from build123d import *

# Parameters (mm, degrees)
F0_W      = 19.05
F0_H      = 19.05
F1_DEPTH  = 19.05
F2_R      = 7.62
F3_DEPTH  = 0.889
F4_R      = 0.999998
F5_DEPTH  = 4.7752
F6_R      = 7.62
F7_DEPTH  = 15.5702
F9_DEPTH  = 6.8573073039
F10_R     = 1.5875
F10_R_2   = 1.9939
F11_DEPTH = 3.4808
F12_R     = 0.999998
F13_DEPTH = 4.7752


with BuildPart() as f1:
    # F0 (on Top) → F1 (new body)
    with BuildSketch(Plane.XY):
        Rectangle(F0_W, F0_H)
    extrude(amount=F1_DEPTH)

    # F2 (on face) → F3 (cut)
    with BuildSketch(Plane.XY.offset(19.05)):
        Circle(F2_R)
        with BuildLine():
            ThreePointArc((4.9464736177, -2.544585921), (-5.5626, 0), (4.9464736177, 2.544585921))
            ThreePointArc((4.9464736177, 2.544585921), (6.5611449159, 1.7206267132), (7.1316849154, 0))
            ThreePointArc((7.1316849154, 0), (6.5611449159, -1.7206267132), (4.9464736177, -2.544585921))
        make_face(mode=Mode.SUBTRACT)
    extrude(amount=-F3_DEPTH, mode=Mode.SUBTRACT)

    # F4 (on face) → F5 (cut)
    with BuildSketch(Plane.XY.offset(19.05)):
        with Locations((-5.7912, -7.874)):
            Circle(F4_R)
        with Locations((5.7912, -7.874)):
            Circle(F4_R)
        with Locations((6.985, 7.747)):
            Circle(F4_R)
        with Locations((-6.985, 7.747)):
            Circle(F4_R)
    extrude(amount=-F5_DEPTH, mode=Mode.SUBTRACT)

    # F6 (on face) → F7 (cut)
    with BuildSketch(Plane.XZ.offset(9.525)):
        with Locations((0, 9.525)):
            Circle(F6_R)
    extrude(amount=-F7_DEPTH, mode=Mode.SUBTRACT)

    # F8 (on face) → F9 (cut, through all)
    with BuildSketch(Plane.XY.offset(19.05)):
        with BuildLine():
            ThreePointArc((4.9464736177, 2.544585921), (-5.5626, 0), (4.9464736177, -2.544585921))
            ThreePointArc((4.9464736177, -2.544585921), (6.5611449159, -1.7206267132), (7.1316849154, 0))
            ThreePointArc((7.1316849154, 0), (6.5611449159, 1.7206267132), (4.9464736177, 2.544585921))
        make_face()
    extrude(amount=-F9_DEPTH, mode=Mode.SUBTRACT)

    # F10 (on face) → F11 (cut, through all)
    with BuildSketch(Plane.XZ.offset(-6.0452)):
        with Locations((0, 9.525)):
            Circle(F10_R)
        with Locations((-4.7752, 9.525)):
            Circle(F10_R_2)
    extrude(amount=-F11_DEPTH, mode=Mode.SUBTRACT)

    # F12 (on face) → F13 (cut)
    with BuildSketch(Plane.XZ.offset(9.525)):
        with Locations((-8.001, 16.51)):
            Circle(F12_R)
        with Locations((8.001, 16.51)):
            Circle(F12_R)
        with Locations((-6.985, 2.54)):
            Circle(F12_R)
        with Locations((6.985, 2.54)):
            Circle(F12_R)
    extrude(amount=-F13_DEPTH, mode=Mode.SUBTRACT)


solid = f1.part
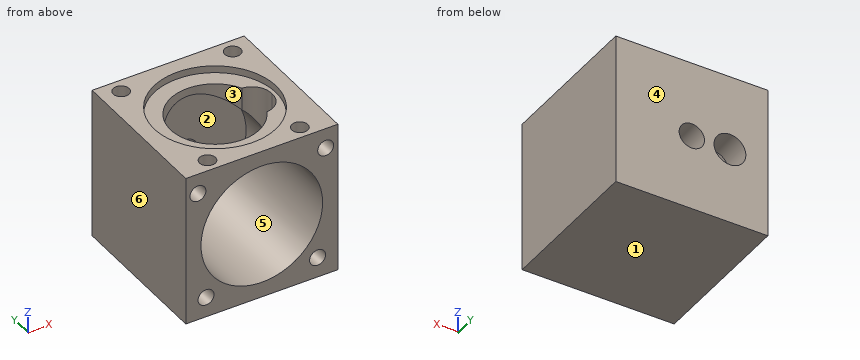
CAD build for the part. Positions are in the model's coordinates, mm. Face numbers are marked on the shaded views. A direction names the side the tool comes from. Give positions to 0.01 mm unless a question says otherwise; leave off trailing zeros. Loops run counter-clockwise (first coordinate to the right, second up) from the corner with the lowest first, then second, coordinate; pieces in that order, holes last. Notation, with made-up numbers: M 12.25,-10.5 L 16.25,-10.5 A14 cw 16.25,2.5 Z; hole C -11,-17.75 d4. An arc over 180 degrees is marked long. One line per question, with ' | ' between items. Start each with the question number.
1. Saw through at D-D on z = 16.51. Give the cut face in (x, y) (3 decimals).
2. Saw through at A-A on x = 0. State how many separate pieces and enclosed holes the cut face has, plus the area to 3 significant figures.
3. 3-axis set-ups, long thin cutter, end or side, ignore diameter. For the marked faces 1, 2 and 3: which of +Z, -Z, +X, -X, +Y, -Y reach the whole face in a straight line?
4. Saw through at C-C on x = 2.25. Give the cut face in (y, z) (3 decimals), plus the area to 3 significant figures.
5. Probe L1, parallel to X at y = 0, z = 16.8 (3 decimals); L2, parallel to Y at x = 0, z = 17.4 (3 decimals); L3, parallel to X at y = -5, z = 1.75 (3 decimals). List the from-to ranges inside material, lowest first. Write a range as from..to.
6. Saw through at B-B on z = 8.5. Give the cut face in (x, y) (3 decimals).
7. Flat gauge pins, fed straight in: pin 1 (1.8 mm diameter, centred on x = 6.985, z = 2.54, fed in from -Y); pin 2 (1.6 mm diameter, centred on x = -6.985, y = 7.747, fed in from +Z); pin 3 (6 mm diameter, centred on x = 1, z = 10, fed in from -Y); pin 4 (2.5 mm diameter, centred on x = -4.78, z = 9.52, fed in from -Y). Where does each tip first touch, or does it go through?
8. Two-plate mould, pull along X, no slides. Class the marked faces 4, 5 and 6: pulls with the +X half, pulls with the -X half, needs draft (parallel to the pull), parting line crosses it, or undercut.
Result sheet:
1) outline: M -9.525,-9.525 L -9.001,-9.525 L -9.001,-4.75 L -7.001,-4.75 L -7.001,-9.525 L -3.045,-9.525 L -3.045,-4.655 A5.563 cw -3.045,4.655 L -3.045,6.045 L 3.045,6.045 L 3.045,4.655 A5.563 cw 4.946,2.545 A2.388 cw 7.132,0 A2.388 cw 4.946,-2.545 A5.563 cw 3.045,-4.655 L 3.045,-9.525 L 7.001,-9.525 L 7.001,-4.75 L 9.001,-4.75 L 9.001,-9.525 L 9.525,-9.525 L 9.525,9.525 L -9.525,9.525 Z; hole C -6.985,7.747 d2; hole C -5.791,-7.874 d2; hole C 5.791,-7.874 d2; hole C 6.985,7.747 d2
2) separate pieces: 3 | enclosed holes: 0 | area: 89.7 mm^2
3) face 1: -Z, +X, -X, +Y, -Y | face 2: -Y | face 3: +Z
4) outline: M -9.525,0 L 9.525,0 L 9.525,19.05 L 7.28,19.05 L 7.28,18.161 L 5.087,18.161 L 5.087,16.805 L 6.045,16.805 L 6.045,2.245 L -9.525,2.245 Z; M -9.525,16.805 L -5.087,16.805 L -5.087,18.161 L -7.28,18.161 L -7.28,19.05 L -9.525,19.05 Z | area: 109 mm^2
5) L1: x = -9.525..-5.563, 7.132..9.525 | L2: y = -9.525..-5.563, 5.563..9.525 | L3: x = -9.525..-7.598, -6.372..6.372, 7.598..9.525
6) outline: M -9.525,-9.525 L -7.551,-9.525 L -7.551,6.045 L -6.485,6.045 L -6.485,9.525 L -9.525,9.525 Z; M -3.065,6.045 L -1.212,6.045 L -1.212,9.525 L -3.065,9.525 Z; M 1.212,6.045 L 7.551,6.045 L 7.551,-9.525 L 9.525,-9.525 L 9.525,9.525 L 1.212,9.525 Z
7) pin 1: stops at y = -4.75 | pin 2: stops at z = 14.27 | pin 3: stops at y = 6.05 | pin 4: passes through
8) face 4: needs draft | face 5: undercut | face 6: pulls with the -X half
